Input: part model. Units: mm. Frame: model coordinates. Give positions to 0.01 mm unless a question says otherwise; leave off trailing zeros. Loops run counter-clockwise (first coordinate to the right, second up) from the corner with the lowest first, then second, coordinate; pieces in that order, holes last. Notation, with made-up numbers: M 56,32 L 78,32 A30 ccw 78,54 Z; hole C 31.25,41.5 d6. An arc over 180 degrees is marked long. Answer as a JSON object with one key per item and string values. Group by question number.
```python
from build123d import *

# Parameters (mm, degrees)
F0_R         = 3.302
F0_R_2       = 1.7
F0_R_3       = 18
F1_DEPTH     = 12.7
F2_SIZE      = 0.508
F3_T1_DEPTH  = 272.9669915773
F4_T4_DEPTH  = 18.4899094878
F4_T10_DEPTH = 18.4899094878
F4_T16_DEPTH = 18.4899094878
F4_T24_DEPTH = 18.4899094878
F4_T30_DEPTH = 18.4899094878
F4_T33_DEPTH = 22.2050244844
F4_T35_DEPTH = 18.4899094878
F4_T37_DEPTH = 37.084


# Not quite as in the source:
# - a fillet or chamfer that OpenCascade refuses, or shapes differently, is made with other operations: its cross-section is extruded or revolved along the edge and cut away or added


with BuildPart() as f1:
    # F0 (on Front) → F1 (new body)
    with BuildSketch(Plane.XZ):
        Polygon((44.9265169831, 0), (44.9265169831, 133.35), (-107.4734830169, 133.35), (-107.4734830169, -102.6728227735), (-89.7620064872, -133.35), (121.9161753795, -133.35), align=None)
        with Locations((-88.4234830169, -76.1876442577)):
            Circle(F0_R, mode=Mode.SUBTRACT)
        with Locations((-88.4234830169, -38.0876442577)):
            Circle(F0_R, mode=Mode.SUBTRACT)
        with Locations((-92.9194827628, 14.6180932346)):
            Circle(F0_R_2, mode=Mode.SUBTRACT)
        with Locations((-69.4244827628, 16.1130932346)):
            Circle(F0_R_2, mode=Mode.SUBTRACT)
        with Locations((-45.9294827628, 14.6180932346)):
            Circle(F0_R_2, mode=Mode.SUBTRACT)
        with Locations((-91.4244827628, 38.1130932346)):
            Circle(F0_R_2, mode=Mode.SUBTRACT)
        with Locations((-69.4244827628, 38.1130932346)):
            Circle(F0_R_3, mode=Mode.SUBTRACT)
        with Locations((-92.9194827628, 61.6080932346)):
            Circle(F0_R_2, mode=Mode.SUBTRACT)
        with Locations((-69.4244827628, 60.1130932346)):
            Circle(F0_R_2, mode=Mode.SUBTRACT)
        with Locations((-47.4244827628, 38.1130932346)):
            Circle(F0_R_2, mode=Mode.SUBTRACT)
        with Locations((-45.9294827628, 61.6080932346)):
            Circle(F0_R_2, mode=Mode.SUBTRACT)
        with Locations((-88.4234830169, 76.2)):
            Circle(F0_R, mode=Mode.SUBTRACT)
        with Locations((-88.4234830169, 114.3)):
            Circle(F0_R, mode=Mode.SUBTRACT)
    extrude(amount=F1_DEPTH)

    # F2
    f2_edges = [f1.edges().sort_by_distance(p)[0] for p in [
        (44.926517, -12.7, 66.675),
        (-31.273483, -12.7, 133.35),
        (-107.473483, -12.7, 15.338589),
        (-98.617745, -12.7, -118.011411),
        (16.077084, -12.7, -133.35),
        (83.421346, -12.7, -66.675),
        (-91.725483, -12.7, -76.187644),
        (-91.725483, -12.7, -38.087644),
        (-94.619483, -12.7, 14.618093),
        (-71.124483, -12.7, 16.113093),
        (-47.629483, -12.7, 14.618093),
        (-93.124483, -12.7, 38.113093),
        (-87.424483, -12.7, 38.113093),
        (-94.619483, -12.7, 61.608093),
        (-71.124483, -12.7, 60.113093),
        (-49.124483, -12.7, 38.113093),
        (-47.629483, -12.7, 61.608093),
        (-91.725483, -12.7, 76.2),
        (-91.725483, -12.7, 114.3),
        (44.926517, 0, 66.675),
        (-31.273483, 0, 133.35),
        (-107.473483, 0, 15.338589),
        (-98.617745, 0, -118.011411),
        (16.077084, 0, -133.35),
        (83.421346, 0, -66.675),
        (-91.725483, 0, -76.187644),
        (-91.725483, 0, -38.087644),
        (-94.619483, 0, 14.618093),
        (-71.124483, 0, 16.113093),
        (-47.629483, 0, 14.618093),
        (-93.124483, 0, 38.113093),
        (-87.424483, 0, 38.113093),
        (-94.619483, 0, 61.608093),
        (-71.124483, 0, 60.113093),
        (-49.124483, 0, 38.113093),
        (-47.629483, 0, 61.608093),
        (-91.725483, 0, 76.2),
        (-91.725483, 0, 114.3),
    ]]
    chamfer(f2_edges, length=F2_SIZE)

    # F3: chamfer of 50.8 on 1 edges, made by hand

    # F3_s2 → F3_t1 (cut)
    with BuildSketch(Plane.XZ.offset(-130.1334957887)):
        Polygon((44.9265169831, 82.55), (-5.8734830169, 133.35), (44.9265169831, 133.35), align=None)
    extrude(amount=F3_T1_DEPTH, mode=Mode.SUBTRACT)

    # F4: fillet of radius 5.08 on 5 edges, made by hand


with BuildPart() as f4_tool2:
    # F4_s3 → F4_t4 (new body)
    with BuildSketch(Plane.XZ.offset(-2.8949547439)):
        with BuildLine():
            ThreePointArc((44.9265169831, 1.3611818976), (45.0996137855, 0.0463811484), (45.6071079319, -1.1788181024))
            Line((45.6071079319, -1.1788181024), (44.9265169831, 0))
            Line((44.9265169831, 0), (44.9265169831, 1.3611818976))
        make_face()
    extrude(amount=F4_T4_DEPTH)

    split(bisect_by=Plane(origin=(22.2092584915, 22.2092584915, 0), x_dir=(0, 0, 1), z_dir=(0.7071067812, 0.7071067812, 0)), keep=Keep.TOP)

    split(bisect_by=Plane(origin=(16.6274734161, 19.1997525055, 9.5998762527), x_dir=(0.755928946, -0.6546536707, 0), z_dir=(-0.6123724357, -0.7071067812, -0.3535533906)), keep=Keep.TOP)


with BuildPart() as f1_1:
    add(f1.part)

    # F4_t1: union F4_tool2
    add(f4_tool2.part)


with BuildPart() as f4_tool8:
    # F4_s9 → F4_t10 (new body)
    with BuildSketch(Plane.XZ.offset(-2.8949547439)):
        with BuildLine():
            ThreePointArc((44.9265169831, 1.3611818976), (45.0996137855, 0.0463811484), (45.6071079319, -1.1788181024))
            Line((45.6071079319, -1.1788181024), (44.9265169831, 0))
            Line((44.9265169831, 0), (44.9265169831, 1.3611818976))
        make_face()
    extrude(amount=F4_T10_DEPTH)

    split(bisect_by=Plane(origin=(22.2092584915, 22.2092584915, 0), x_dir=(0, 0, 1), z_dir=(-0.7071067812, -0.7071067812, 0)), keep=Keep.TOP)

    split(bisect_by=Plane(origin=(16.6274734161, 19.1997525055, 9.5998762527), x_dir=(-0.755928946, 0.6546536707, 0), z_dir=(0.6123724357, 0.7071067812, 0.3535533906)), keep=Keep.TOP)


with BuildPart() as f1_2:
    add(f1_1.part)

    # F4_t7: union F4_tool8
    add(f4_tool8.part)


with BuildPart() as f4_tool14:
    # F4_s15 → F4_t16 (new body)
    with BuildSketch(Plane.XZ.offset(-2.8949547439)):
        with BuildLine():
            ThreePointArc((44.9265169831, 1.3611818976), (45.0996137855, 0.0463811484), (45.6071079319, -1.1788181024))
            Line((45.6071079319, -1.1788181024), (44.9265169831, 0))
            Line((44.9265169831, 0), (44.9265169831, 1.3611818976))
        make_face()
    extrude(amount=F4_T16_DEPTH)

    split(bisect_by=Plane(origin=(22.2092584915, 22.2092584915, 0), x_dir=(0, 0, 1), z_dir=(-0.7071067812, -0.7071067812, 0)), keep=Keep.TOP)

    split(bisect_by=Plane(origin=(28.5592584915, -28.5592584915, 0), x_dir=(0, 0, 1), z_dir=(-0.7071067812, 0.7071067812, 0)), keep=Keep.TOP)

    split(bisect_by=Plane(origin=(16.6274734161, 19.1997525055, 9.5998762527), x_dir=(0.755928946, -0.6546536707, 0), z_dir=(-0.6123724357, -0.7071067812, -0.3535533906)), keep=Keep.TOP)

    split(bisect_by=Plane(origin=(22.1267347301, -25.5497525055, 12.7748762527), x_dir=(-0.755928946, -0.6546536707, 0), z_dir=(-0.6123724357, 0.7071067812, -0.3535533906)), keep=Keep.TOP)


with BuildPart() as f1_3:
    add(f1_2.part)

    # F4_t13: union F4_tool14
    add(f4_tool14.part)


with BuildPart() as f4_tool22:
    # F4_s23 → F4_t24 (new body)
    with BuildSketch(Plane.XZ.offset(-2.8949547439)):
        with BuildLine():
            ThreePointArc((44.9265169831, 1.3611818976), (45.0996137855, 0.0463811484), (45.6071079319, -1.1788181024))
            Line((45.6071079319, -1.1788181024), (44.9265169831, 0))
            Line((44.9265169831, 0), (44.9265169831, 1.3611818976))
        make_face()
    extrude(amount=F4_T24_DEPTH)

    split(bisect_by=Plane(origin=(28.5592584915, -28.5592584915, 0), x_dir=(0, 0, 1), z_dir=(0.7071067812, -0.7071067812, 0)), keep=Keep.TOP)

    split(bisect_by=Plane(origin=(22.1267347301, -25.5497525055, 12.7748762527), x_dir=(-0.755928946, -0.6546536707, 0), z_dir=(-0.6123724357, 0.7071067812, -0.3535533906)), keep=Keep.TOP)


with BuildPart() as f1_4:
    add(f1_3.part)

    # F4_t21: union F4_tool22
    add(f4_tool22.part)


with BuildPart() as f4_tool28:
    # F4_s29 → F4_t30 (new body)
    with BuildSketch(Plane.XZ.offset(-2.8949547439)):
        with BuildLine():
            ThreePointArc((44.9265169831, 1.3611818976), (45.0996137855, 0.0463811484), (45.6071079319, -1.1788181024))
            Line((45.6071079319, -1.1788181024), (44.9265169831, 0))
            Line((44.9265169831, 0), (44.9265169831, 1.3611818976))
        make_face()
    extrude(amount=F4_T30_DEPTH)

    split(bisect_by=Plane(origin=(28.5592584915, -28.5592584915, 0), x_dir=(0, 0, 1), z_dir=(-0.7071067812, 0.7071067812, 0)), keep=Keep.TOP)

    split(bisect_by=Plane(origin=(22.1267347301, -25.5497525055, 12.7748762527), x_dir=(0.755928946, 0.6546536707, 0), z_dir=(0.6123724357, -0.7071067812, 0.3535533906)), keep=Keep.TOP)


with BuildPart() as f1_5:
    add(f1_4.part)

    # F4_t27: union F4_tool28
    add(f4_tool28.part)

    # F4_s34 → F4_t33 (cut)
    with BuildSketch(Plane.XZ.offset(-4.7525122422)):
        with BuildLine():
            ThreePointArc((44.9265169831, 80.4457951032), (44.5398250082, 82.3898269396), (43.4386194315, 84.0378975516))
            Line((43.4386194315, 84.0378975516), (44.9265169831, 82.55))
            Line((44.9265169831, 82.55), (44.9265169831, 80.4457951032))
        make_face()
        with BuildLine():
            ThreePointArc((-4.3855854653, 131.8621024484), (-6.0336560773, 132.9633080252), (-7.9776879138, 133.35))
            Line((-7.9776879138, 133.35), (-5.8734830169, 133.35))
            Line((-5.8734830169, 133.35), (-4.3855854653, 131.8621024484))
        make_face()
    extrude(amount=F4_T33_DEPTH, mode=Mode.SUBTRACT)

    # F4_s36 → F4_t35 (cut)
    with BuildSketch(Plane.XZ.offset(-2.8949547439)):
        with BuildLine():
            ThreePointArc((-107.4734830169, -101.3116408759), (-107.3003862145, -102.626441625), (-106.7928920681, -103.8516408759))
            Line((-106.7928920681, -103.8516408759), (-107.4734830169, -102.6728227735))
            Line((-107.4734830169, -102.6728227735), (-107.4734830169, -101.3116408759))
        make_face()
    extrude(amount=F4_T35_DEPTH, mode=Mode.SUBTRACT)

    # F4_s38 → F4_t37 (cut)
    with BuildSketch(Plane.XZ.offset(-12.192)):
        with BuildLine():
            ThreePointArc((-107.4734830169, 128.27), (-105.9855854653, 131.8621024484), (-102.3934830169, 133.35))
            Line((-102.3934830169, 133.35), (-107.4734830169, 133.35))
            Line((-107.4734830169, 133.35), (-107.4734830169, 128.27))
        make_face()
    extrude(amount=F4_T37_DEPTH, mode=Mode.SUBTRACT)


solid = f1_5.part
```
1. Section A-A (z = 76.2). Output: boundary loops of the cut face in (x, y).
2. Section D-D (z = 114.3). Output: boundary loops of the cut face in (x, y).
3. Section C-C (x = 79.5). Output: boundary loops of the cut face in (y, z), then the cut area to 3 significant figures.
4. Material intervals for L1, parallel to Z at x = -69.5, y = -7.5; L2, parallel to Z at x = -69, y = -4; L3, parallel to X at y = -7, z = 7.5, sorted ascending.
5. First-contact query: P1, Ø5.5, axis at x = -47.42, z = 38.11, coming from the +Y side; P2, Ø7.5, axis at x = -88.42, z = -38.09, coming from the +Y side; P3, Ø3, axis at y = -8.5, z = -5, coming from the +X side; P4, Ø1, axis at y = -10.5, z = 47, coming from the +X side. Flat tips, straight axial feed; report the tip coordinate or a pass-through.
6. Section B-B (y = -2.75). Count the separate pieces of the cut face and the enclosed holes in it, then the cut area to 3 significant figures.
7. Mould query, pull axis X, two halves, no side actions, for faces 1 (the flat face through (15, -6, -133.35)), 2 (the cylindrical face through (-86.648, -6.268, 117.084)), 3 (the cylindrical face through (-87.407, -6.268, 38.905)), 4 (the flat face through (19.861, -6.261, 107.615)). Classes: pulls with the +X half, pulls with the -X half, needs draft (parallel to the pull), parting line crosses it, or undercut.
Geometry results:
{
 "1": {"outline": "M -107.47,-12.19 L -106.97,-12.7 L -92.23,-12.7 L -91.73,-12.19 L -91.73,-0.51 L -92.23,0 L -106.97,0 L -107.47,-0.51 Z; M -85.12,-12.19 L -84.61,-12.7 L 44.42,-12.7 L 44.93,-12.19 L 44.93,-0.51 L 44.42,0 L -84.61,0 L -85.12,-0.51 Z"},
 "2": {"outline": "M -107.47,-12.19 L -106.97,-12.7 L -92.23,-12.7 L -91.73,-12.19 L -91.73,-0.51 L -92.23,0 L -106.97,0 L -107.47,-0.51 Z; M -85.12,-12.19 L -84.61,-12.7 L 13.18,-12.7 L 13.18,0 L -84.61,0 L -85.12,-0.51 Z"},
 "3": {"outline": "M -12.7,-132.84 L -12.19,-133.35 L -0.51,-133.35 L 0,-132.84 L 0,-60.9 L -0.51,-59.88 L -12.19,-59.88 L -12.7,-60.9 Z", "area": "932 mm2"},
 "4": {"L1": "-133.35 to 14.41, 17.81 to 20.11, 56.11 to 58.41, 61.81 to 133.35", "L2": "-133.35 to 14.47, 17.76 to 20.12, 56.11 to 58.47, 61.76 to 133.35", "L3": "-107.47 to 44.93"},
 "5": {"P1": "y = 0", "P2": "y = -0.06", "P3": "x = 48.68", "P4": "x = 44.93"},
 "6": {"separate pieces": "1", "enclosed holes": "13", "area": "43,000 mm2"},
 "7": {"face 1": "needs draft", "face 2": "undercut", "face 3": "undercut", "face 4": "pulls with the +X half"}
}
